For this review, take the finished solid that the model builds, in its own axes (mm). Face numbers are marked on the shaded views. A direction names the side the tool comes from. Coordinates: 2 decimals unless noted, no trailing zeros. One line per item, written item: value. Start each with the question number.
(1) Clearance check with flat-ended pins moving along their axes: pin 1 (9 mm diameter, centred on x = 3, y = -4.5, fed in from +Z); pin 2 (1.5 mm diameter, centred on x = 12, z = 28.5, fed in from -Y); pin 3 (2 mm diameter, centred on y = -10.5, z = 10.5, fed in from -X). State where each tip first meets the part, or that it passes through.
(2) Mouldability with a two-part tool opening along Y and no side actions: class the marked faces 6, 7 and 8 as released by +Y, released by -Y, zero draft, split by the parting line, or undercut.
(3) For the marked faces 1, 2, 3, 4 and 5, list the 3-axis set-ups (+Z, -Z, +X, -X, +Y, -Y) from which the entire face can be reached by the end or side of a thin tool; tool diameter is ignored.
(4) Consider section A-A on y = 4. Count the separate pieces of the cut face and the enclosed holes in it, then the cut area to 3 significant figures.
(5) To check wall thickness, follow line 1 along Y through (x, z) = (0, 9); line 2 along Y through (x, z) = (0, 10); line 3 along Z through (x, y) = (-1, 8). State the ranges of each line that lie inside material, in increasing order.
```python
from build123d import *

# Parameters (mm, degrees)
ESQUISSE1_R                   = 21
ESQUISSE1_R_2                 = 3.25
BOSS_EXTRU_1_DEPTH            = 31
ESQUISSE2_R                   = 21
ESQUISSE2_R_2                 = 15
BOSS_EXTRU_2_DEPTH            = 6
ENL_V_MAT_EXTRU_9_DEPTH       = 12
CHANFREIN1_SIZE               = 1
ESQUISSE11_R                  = 1.25
ENL_V_MAT_EXTRU_10_DEPTH      = 48.444704657
ESQUISSE12_R                  = 4.25
ENL_V_MAT_EXTRU_11_DEPTH      = 4
ENL_V_MAT_EXTRU_12_DEPTH      = 56.054580282
ENL_V_MAT_EXTRU_12_DEPTH_BACK = 56.054580282
ESQUISSE13_R                  = 1.75


with BuildPart() as part:
    # Esquisse1 → Boss.-Extru.1 (new body)
    with BuildSketch(Plane.XY):
        Circle(ESQUISSE1_R)
        Circle(ESQUISSE1_R_2, mode=Mode.SUBTRACT)
    extrude(amount=BOSS_EXTRU_1_DEPTH)

    # Esquisse2 → Boss.-Extru.2 (add)
    with BuildSketch(Plane.XY.offset(31)):
        Circle(ESQUISSE2_R)
        Circle(ESQUISSE2_R_2, mode=Mode.SUBTRACT)
    extrude(amount=BOSS_EXTRU_2_DEPTH)

    # Esquisse9 → Enlèv. mat.-Extru.9 (cut)
    with BuildSketch(Plane.XY.offset(31)):
        Polygon((11.35, -6.552925555), (11.35, 6.552925555), (0, 13.105851111), (-11.35, 6.552925555), (-11.35, -6.552925555), (0, -13.105851111), align=None)
    extrude(amount=-ENL_V_MAT_EXTRU_9_DEPTH, mode=Mode.SUBTRACT)

    # Chanfrein1
    chanfrein1_edges = [part.edges().sort_by_distance(p)[0] for p in [
        (-15, 0, 37),
    ]]
    chamfer(chanfrein1_edges, length=CHANFREIN1_SIZE)

    # Esquisse10 → Enlèvement de matière-Révolution1 (revolve, cut)
    with BuildSketch(Plane(origin=(0, 0, 0), x_dir=(0, 0, -1), z_dir=(1, 0, 0)), mode=Mode.PRIVATE) as enl_vement_de_mati_re_r_volution1_sk:
        with BuildLine():
            Line((-35, 21), (-2, 21))
            Line((-2, 21), (-3, 17))
            ThreePointArc((-3, 17), (-18.5, 17.5), (-34, 17))
            Line((-34, 17), (-35, 21))
        make_face()
    revolve(enl_vement_de_mati_re_r_volution1_sk.sketch.rotate(Axis((0, 0, 0), (0, 0, 1)), 90), axis=Axis((0, 0, 0), (0, 0, 1)), mode=Mode.SUBTRACT)

    # Esquisse11 → Enlèv. mat.-Extru.10 (cut, through all)
    with BuildSketch(Plane(origin=(0, 0, 0), x_dir=(-1, 0, 0), z_dir=(0, 0, -1))):
        with Locations((-6.92820323, 4)):
            Circle(ESQUISSE11_R)
        with Locations((6.92820323, 4)):
            Circle(ESQUISSE11_R)
        with Locations((0, -8)):
            Circle(ESQUISSE11_R)
    extrude(amount=-ENL_V_MAT_EXTRU_10_DEPTH, mode=Mode.SUBTRACT)

    # Esquisse12 → Enlèv. mat.-Extru.11 (cut)
    with BuildSketch(Plane(origin=(0, 0, 0), x_dir=(-1, 0, 0), z_dir=(0, 0, -1))):
        with Locations((-6.92820323, 4)):
            Circle(ESQUISSE12_R)
        with Locations((6.92820323, 4)):
            Circle(ESQUISSE12_R)
        with Locations((0, -8)):
            Circle(ESQUISSE12_R)
    extrude(amount=-ENL_V_MAT_EXTRU_11_DEPTH, mode=Mode.SUBTRACT)

    # Esquisse13 → Enlèv. mat.-Extru.12 (cut, two sides: drawn at the far end of the back side and taken through both)
    with BuildSketch(Plane(origin=(-5.675, -9.829388333, 0), x_dir=(0.8660254037844387, -0.49999999999999983, 0), z_dir=(0.49999999999999983, 0.8660254037844387, 0)).offset(-ENL_V_MAT_EXTRU_12_DEPTH_BACK)):
        with Locations(Location((0, -25, 0), (0, 0, 180))):
            Circle(ESQUISSE13_R)
        with Locations(Location((0, -10, 0), (0, 0, 180))):
            Circle(ESQUISSE13_R)
    extrude(amount=ENL_V_MAT_EXTRU_12_DEPTH + ENL_V_MAT_EXTRU_12_DEPTH_BACK, mode=Mode.SUBTRACT)


solid = part.part
```
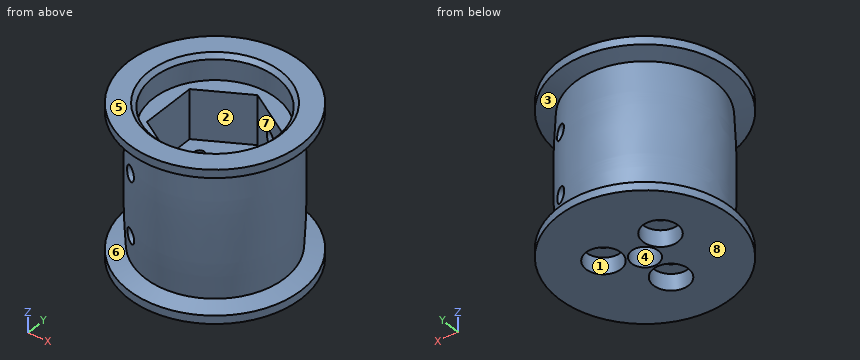
Geometry check:
1. pin 1: stops at z = 19
1. pin 2: stops at y = -13.13
1. pin 3: stops at x = -14.54
2. face 6: split by the parting line
2. face 7: undercut
2. face 8: zero draft
3. face 1: -Z
3. face 2: +Z
3. face 3: none
3. face 4: +Z, -Z
3. face 5: +Z, +X, -X, +Y, -Y
4. separate pieces: 3
4. enclosed holes: 1
4. area: 684 mm^2
5. line 1: y = -17.31 to -9.25, -6.75 to -3.25, 3.25 to 17.31
5. line 2: y = -17.35 to -9.25, -6.75 to -3.5, 3.5 to 17.35
5. line 3: z = 0 to 19
